from build123d import *

# Parameters (mm, degrees)
SKETCH1_W                  = 30
SKETCH1_H                  = 38
BOSS_EXTRUDE1_DEPTH        = 3
SKETCH2_R                  = 5
CUT_EXTRUDE1_DEPTH         = 3
SKETCH6_W                  = 10
SKETCH6_H                  = 3
CUT_EXTRUDE2_DEPTH         = 3
CUT_EXTRUDE3_DEPTH         = 3
SKETCH9_W                  = 10
SKETCH9_H                  = 3
CUT_EXTRUDE5_DEPTH         = 10
CUT_EXTRUDE6_DEPTH         = 10
M2_5_CLEARANCE_SLOT1_DEPTH = 3
SKETCH17_W                 = 10
SKETCH17_H                 = 10
CUT_EXTRUDE7_DEPTH         = 10
FILLET1_R                  = 1


# Read off the part's stored shape, not the designer's step: M2.5 Clearance Slot1
with BuildPart() as part:
    # Sketch1 → Boss-Extrude1 (new body)
    with BuildSketch(Plane(origin=(0, 0, 0), x_dir=(0, 0, -1), z_dir=(1, 0, 0))):
        with Locations((15, 19)):
            Rectangle(SKETCH1_W, SKETCH1_H)
    extrude(amount=BOSS_EXTRUDE1_DEPTH)

    # Sketch2 → Cut-Extrude1 (cut)
    with BuildSketch(Plane(origin=(3, 0, 0), x_dir=(0, 0, -1), z_dir=(1, 0, 0))):
        with Locations((20, 18)):
            Circle(SKETCH2_R)
    extrude(amount=-CUT_EXTRUDE1_DEPTH, mode=Mode.SUBTRACT)

    # Sketch6 → Cut-Extrude2 (cut)
    with BuildSketch(Plane(origin=(3, 0, 0), x_dir=(0, 0, -1), z_dir=(1, 0, 0))):
        with Locations((5, 1.5)):
            Rectangle(SKETCH6_W, SKETCH6_H)
        with Locations((25, 1.5)):
            Rectangle(SKETCH6_W, SKETCH6_H)
    extrude(amount=-CUT_EXTRUDE2_DEPTH, mode=Mode.SUBTRACT)

    # Sketch7 → Cut-Extrude3 (cut)
    with BuildSketch(Plane(origin=(3, 0, 0), x_dir=(0, 0, -1), z_dir=(1, 0, 0))):
        Polygon((3, 3), (3, 5.9), (1.6, 5.9), (1.6, 8.6), (3, 8.6), (3, 10.3), (6.1, 10.3), (6.1, 8.6), (7.5, 8.6), (7.5, 5.9), (6.1, 5.9), (6.1, 3), align=None)
    extrude(amount=-CUT_EXTRUDE3_DEPTH, mode=Mode.SUBTRACT)

    # Sketch9 → Cut-Extrude5 (cut)
    with BuildSketch(Plane(origin=(3, 0, 0), x_dir=(0, 0, -1), z_dir=(1, 0, 0))):
        with Locations((5, 36.5)):
            Rectangle(SKETCH9_W, SKETCH9_H)
        with Locations((25, 36.5)):
            Rectangle(SKETCH9_W, SKETCH9_H)
    extrude(amount=-CUT_EXTRUDE5_DEPTH, mode=Mode.SUBTRACT)

    # Sketch12 → Cut-Extrude6 (cut)
    with BuildSketch(Plane(origin=(3, 0, 0), x_dir=(0, 0, -1), z_dir=(1, 0, 0))):
        Polygon((6.6, 35), (6.6, 32.1), (8, 32.1), (8, 29.4), (6.6, 29.4), (6.6, 27.7), (3.5, 27.7), (3.5, 29.4), (2.1, 29.4), (2.1, 32.1), (3.5, 32.1), (3.5, 35), align=None)
    extrude(amount=-CUT_EXTRUDE6_DEPTH, mode=Mode.SUBTRACT)

    # M2.5 Clearance Slot1 outline → M2.5 Clearance Slot1 (cut)
    with BuildSketch(Plane.YZ):
        with BuildLine():
            Line((11.4, -22.05), (11.4, -17.95))
            ThreePointArc((11.4, -17.95), (9.95, -16.5), (8.5, -17.95))
            Line((8.5, -17.95), (8.5, -22.05))
            ThreePointArc((8.5, -22.05), (9.95, -23.5), (11.4, -22.05))
        make_face()
        with BuildLine():
            Line((27.5, -22.05), (27.5, -17.95))
            ThreePointArc((27.5, -17.95), (26.05, -16.5), (24.6, -17.95))
            Line((24.6, -17.95), (24.6, -22.05))
            ThreePointArc((24.6, -22.05), (26.05, -23.5), (27.5, -22.05))
        make_face()
    extrude(amount=M2_5_CLEARANCE_SLOT1_DEPTH, mode=Mode.SUBTRACT)

    # Sketch17 → Cut-Extrude7 (cut)
    with BuildSketch(Plane(origin=(3, 0, 0), x_dir=(0, 0, -1), z_dir=(1, 0, 0))):
        with Locations((25, 18)):
            Rectangle(SKETCH17_W, SKETCH17_H)
    extrude(amount=-CUT_EXTRUDE7_DEPTH, mode=Mode.SUBTRACT)

    # Fillet1
    fillet1_edges = [part.edges().sort_by_distance(p)[0] for p in [
        (1.5, 23, -30),
        (1.5, 13, -30),
    ]]
    fillet(fillet1_edges, radius=FILLET1_R)


solid = part.part
Check sheet for the modelled part. Datum: model origin and axes. Units: mm. A direction names the side the tool comes from. Give positions to 0.01 mm unless a question says otherwise; leave off trailing zeros. Loops run counter-clockwise (first coordinate to the right, second up) from the corner with the lowest first, then second, coordinate; pieces in that order, holes last. Notation, with made-up numbers: M -28,-25.75 L -15,-25.75 A19 ccw -15,1.25 Z; hole C 19,24 d2. An arc over 180 degrees is marked long. Use a Markdown table: item, result. Add a question column.
Q1. Sectioned sample at A-A, the plane y = 5.5. Record the cut outline in (x, z), then the cut area to 3 significant figures.
Q2. Go/stop test with flat-tipped pins: pin 1 (1.5 mm diameter, centred on x = 1, z = -23.5, fed in from -Y); pin 2 (1.5 mm diameter, centred on x = 1, z = -4.5, fed in from +Y); pin 3 (0.9 mm diameter, centred on x = 1, y = 1.5, fed in from +Z). Record where each tip stops, or that it passes through.
Q3. Tool access check on faces 5 (the cylindrical face through (1.479, 12.715, -29.699)), 6 (the flat face through (2, 4, -3)), 7 (the flat face through (2, 3, -25)), 8 (the flat face through (2, 27.7, -5)), 9 (the cylindrical face through (1.5, 9.9, -23.5)). Record the directions out of +Z, -Z, +X, -X, +Y, -Y that give a thin tool (end or side, any length) a straight path to the whole face; none if there is none.
Q4. Sectioned sample at C-C, the plane x = 0.75. Give the number of separate pieces and of enclosed holes in the cut face, then the cut area to 3 significant figures.
Q5. Sectioned sample at D-D, the plane y = 31. Record the cut outline in (x, z), then the cut area to 3 significant figures.
Q6. Scan lines: line 1 along Y through (x, z) = (2.5, -22); line 2 along Y through (x, z) = (2.75, -26.25); line 3 along Z through (x, y) = (0.55, 34.5). Record each from-to range of solid material in increasing order. Write a range as [from, to].
Q7. Sectioned sample at B-B, the plane z = -19. Record the cut outline in (x, y).
Q8. Mould release check, pull along Z, two halves, no side actions. Record for faces 1 (the flat face through (2, 1, -10)), 2 (the flat face through (0, 19.3, -14.8)), 3 (the flat face through (2, 9, -3)), 4 (the flat face through (1, 7, -30)): pulls with the +Z half, pulls with the -Z half, needs draft (parallel to the pull), parting line crosses it, or undercut.
Verdict:
| question | item | result |
|---|---|---|
| 1 | outline | M 0,-30 L 3,-30 L 3,-6.1 L 0,-6.1 Z; M 0,-3 L 3,-3 L 3,0 L 0,0 Z |
| 1 | area | 80.7 mm^2 |
| 2 | pin 1 | y = 3 |
| 2 | pin 2 | y = 27.7 |
| 2 | pin 3 | z = -10 |
| 3 | face 5 | -Z, +X, -X |
| 3 | face 6 | +X, -X, -Y |
| 3 | face 7 | -Z, +X, -X, -Y |
| 3 | face 8 | +X, -X, +Y |
| 3 | face 9 | +X, -X |
| 4 | separate pieces | 1 |
| 4 | enclosed holes | 2 |
| 4 | area | 783 mm^2 |
| 5 | outline | M 0,-30 L 3,-30 L 3,-8 L 0,-8 Z; M 0,-2.1 L 3,-2.1 L 3,0 L 0,0 Z |
| 5 | area | 72.3 mm^2 |
| 6 | line 1 | [3, 8.5], [11.4, 13], [23, 24.6], [27.5, 35] |
| 6 | line 2 | [3, 13], [23, 35] |
| 6 | line 3 | [-30, -6.6], [-3.5, 0] |
| 7 | outline | M 0,0 L 3,0 L 3,8.5 L 0,8.5 Z; M 0,11.4 L 3,11.4 L 3,13.1 L 0,13.1 Z; M 0,22.9 L 3,22.9 L 3,24.6 L 0,24.6 Z; M 0,27.5 L 3,27.5 L 3,38 L 0,38 Z |
| 8 | face 1 | pulls with the +Z half |
| 8 | face 2 | needs draft |
| 8 | face 3 | undercut |
| 8 | face 4 | pulls with the -Z half |
